Source: CAD feature listing. Evaluate the final solid. Frame: model axes, mm. A direction names the side the tool comes from. Coordinates: 2 decimals unless noted, no trailing zeros. Order: outer loops, then holes, each group sorted by start corner. A loop starts at its lowest first (then second) coordinate and runs counter-clockwise, first axis right, second up.
```python
from build123d import *

# Parameters (mm, degrees)
SKETCH2_R             = 5.5
CUT_EXTRUDE1_DEPTH    = 0.1
CUT_EXTRUDE2_DEPTH    = 0.1
CORTAR_EXTRUIR1_START = -0.25
CROQUIS1_R            = 5.5
CORTAR_EXTRUIR1_DEPTH = 0.25
FILLET1_R             = 0.5
SKETCH4_W             = 0.4
SKETCH4_H             = 6


with BuildPart() as part:
    # Sketch1 → Revolve1 (revolve)
    with BuildSketch(Plane.XY):
        with BuildLine():
            Line((8, 25), (0, 25))
            Line((0, 25), (0, 0))
            Line((0, 0), (8, 0))
            ThreePointArc((8, 0), (8.092932458, 0.406232629), (7.928060317, 0.788957816))
            ThreePointArc((7.928060317, 0.788957816), (7.803725589, 0.995469347), (7.760416667, 1.232599004))
            Line((7.760416667, 1.232599004), (7.760416667, 1.642400996))
            ThreePointArc((7.760416667, 1.642400996), (7.791064683, 1.842850794), (7.880208333, 2.024984899))
            ThreePointArc((7.880208333, 2.024984899), (7.969351983, 2.207119004), (8, 2.407568802))
            Line((8, 2.407568802), (8, 25))
        make_face()
    revolve(axis=Axis((0, 25, 0), (0, -1, 0)))

    # Sketch2 → Cut-Extrude1 (cut)
    with BuildSketch(Plane(origin=(0, 25, 0), x_dir=(-1, 0, 0), z_dir=(0, 1, 0))):
        with Locations(Location((0, 0, 0), (0, 0, 270))):
            Circle(SKETCH2_R)
    extrude(amount=-CUT_EXTRUDE1_DEPTH, mode=Mode.SUBTRACT)

    # Sketch3 → Cut-Extrude2 (cut)
    with BuildSketch(Plane(origin=(0, 24.9, 0), x_dir=(-1, 0, 0), z_dir=(0, 1, 0))):
        with BuildLine():
            Line((-5.499090834, -0.1), (-0.1, -0.1))
            Line((-0.1, -0.1), (-0.1, -5.499090834))
            ThreePointArc((-0.1, -5.499090834), (-0.050002066, -5.499772704), (0, -5.5))
            ThreePointArc((0, -5.5), (0.050002066, -5.499772704), (0.1, -5.499090834))
            Line((0.1, -5.499090834), (0.1, -0.1))
            Line((0.1, -0.1), (5.499090834, -0.1))
            ThreePointArc((5.499090834, -0.1), (5.499772704, -0.050002066), (5.5, 0))
            ThreePointArc((5.5, 0), (5.499772704, 0.050002066), (5.499090834, 0.1))
            Line((5.499090834, 0.1), (0.1, 0.1))
            Line((0.1, 0.1), (0.1, 5.499090834))
            ThreePointArc((0.1, 5.499090834), (0.050002066, 5.499772704), (0, 5.5))
            ThreePointArc((0, 5.5), (-0.050002066, 5.499772704), (-0.1, 5.499090834))
            Line((-0.1, 5.499090834), (-0.1, 0.1))
            Line((-0.1, 0.1), (-5.499090834, 0.1))
            ThreePointArc((-5.499090834, 0.1), (-5.499772704, 0.050002066), (-5.5, 0))
            ThreePointArc((-5.5, 0), (-5.499772704, -0.050002066), (-5.499090834, -0.1))
        make_face()
    extrude(amount=-CUT_EXTRUDE2_DEPTH, mode=Mode.SUBTRACT)

    # Croquis1 → Cortar-Extruir1 (cut)
    with BuildSketch(Plane.XZ.offset(CORTAR_EXTRUIR1_START)):
        with Locations(Location((0, 0, 0), (0, 0, 88.95820115))):
            Circle(CROQUIS1_R)
    extrude(amount=CORTAR_EXTRUIR1_DEPTH, mode=Mode.SUBTRACT)

    # Fillet1
    fillet1_edges = [part.edges().sort_by_distance(p)[0] for p in [
        (-8, 25, 0),
        (-8, 0, 0),
    ]]
    fillet(fillet1_edges, radius=FILLET1_R)

    # Sketch4 → Revolución1 (revolve)
    with BuildSketch(Plane(origin=(0, 0, 0), x_dir=(-1, 0, 0), z_dir=(0, 0, -1)), mode=Mode.PRIVATE) as revoluci_n1_sk:
        with Locations((-3.941657387, -2.75)):
            Rectangle(SKETCH4_W, SKETCH4_H)
    revoluci_n1 = revolve(revoluci_n1_sk.sketch.rotate(Axis((3.741657387, -5.75, 0), (0, 1, 0)), 90), axis=Axis((3.741657387, -5.75, 0), (0, 1, 0)))

    # Simetría1: Revolución1 across plane
    add(revoluci_n1.mirror(Plane(origin=(0, 0, 0), x_dir=(0, 0, 1), z_dir=(1, 0, 0))))


solid = part.part
```
1. Section query A-A on y = 3. Return loops of the section in (x, z), plus the area to 3 significant figures.
Findings:
outline: circle Ø16 at (0, 0)
area: 201 mm2
2. Pin query (flat end, axial travel): P1, Ø4, axis at x = -4.5, z = -0.5, coming from the +Y side; P2, Ø1.5, axis at y = 8, z = 0.5, coming from the -X side; P3, Ø2, axis at y = 6.5, z = 3.5, coming from the +X side; P4, Ø5, axis at y = 16, z = 4, coming from the +X side. Return the tip coordinate at first contact, or that it passes through.
Findings:
P1: stops at y = 25
P2: stops at x = -8
P3: stops at x = 7.6
P4: stops at x = 7.86
3. Section query B-B on y = -3.5. Return loops of the section in (x, z), plus the area to 3 significant figures.
Findings:
outline: circle Ø0.8 at (-3.74, 0); circle Ø0.8 at (3.74, 0)
area: 1.01 mm2
4. Ray query, line 1 (X direction, y = 0.15, z = 0) (3 decimals); line 2 (Y direction, x = 0, z = -7.25); line 3 (Z direction, x = 0, y = 0.15) (3 decimals). Return the intervals inside material, ascending.
Findings:
line 1: x = -7.875 to -5.5, -4.142 to -3.342, 3.342 to 4.142, 5.5 to 7.875
line 2: y = 0 to 25
line 3: z = -7.875 to -5.5, 5.5 to 7.875
5. Access query for faces 1 (the face through (-1.682, 1.44, -7.576)), 2 (the face through (0, 0.25, 0)), 3 (the face through (2, 24.9, 2)). Directions: +Z, -Z, +X, -X, +Y, -Y. A direction counts if a zero-diameter tool reaches every point of the face in a straight line with its end or side. Return the directions, or none.
Findings:
face 1: none
face 2: -Y
face 3: +Y
6. Draft query along X for faces 4 (the face through (-2, 24.9, -2)), 5 (the face through (-4, 25, 4)), 6 (the face through (-1.73, 13.61, -7.81)). Return one class per face: released by +X, released by -X, zero draft, split by the parting line, or undercut.
Findings:
face 4: undercut
face 5: zero draft
face 6: split by the parting line
